Check sheet for the modelled part. Datum: model origin and axes. Units: mm. A direction names the side the tool comes from. Round coordinates to 2 decimals unless told otherwise and drop trailing zeros. Write each loop counter-clockwise with the first axis right and the second up, starting at its lowest first coordinate (ties: lowest second). Pieces come first, ordered by that corner, then holes.
Item 1: Release check for a two-part mould opening along X. For faces 1 (the flat face through (11, 143.002, 0)), 2 (the flat face through (34.355, 156.823, 9.392)), 3 (the flat face through (24, 143.002, 0)), 4 (the flat face through (18, 157, -19.05)) record: +X half, -X half, draft (parallel to the pull), parting line (faces both ways), or undercut.
Item 2: Tool access check on faces 5 (the flat face through (34.2, 156.82, -9.66)), 6 (the flat face through (31, 154.305, -8)). Record the directions out of +Z, -Z, +X, -X, +Y, -Y that give a thin tool (end or side, any length) a straight path to the whole face; none if there is none.
Item 3: Cross-section at B-B on y = 146.75. Enter the section's corners in (x, z), plus the area to 3 significant figures.
Item 4: Go/stop test with flat-tipped pins: pin 1 Ø6 at (x, y) = (4, 146.5) entering from -Z; pin 2 Ø4 at (x, y) = (6.5, 152) entering from -Z; pin 3 Ø6 at (x, y) = (3, 147) entering from -Z. Record where each tip stops, or that it passes through.
Item 5: Cross-section at A-A on x = 17.78. Enter the section's corners in (y, z) (3 decimals).
Item 6: Material ranges on line 1 (Y direction, x = 1, z = -1) (3 decimals); line 2 (Z direction, x = 24.13, y = 142.95); line 3 (X direction, y = 147.5, z = -8), recorded low to high.
from build123d import *

# Parameters (mm, degrees)
PAD012_DEPTH    = 5.08
SKETCH059_R     = 15.24
PAD013_DEPTH    = 11.43
SKETCH065_R     = 3.20675
POCKET010_DEPTH = 0.127


with BuildPart() as part:
    # Sketch058 → Pad012 (new body)
    with BuildSketch(Plane.XZ):
        Polygon((21.997045, 0), (10.998523, 19.05), (-10.998523, 19.05), (-21.997045, 0), (-10.998523, -19.05), (10.998523, -19.05), align=None)
    extrude(amount=PAD012_DEPTH)

    # Sketch059 (on Face8 of Pad012) → Pad013 (join)
    with BuildSketch(Plane.XZ.offset(5.08)):
        Circle(SKETCH059_R)
    extrude(amount=PAD013_DEPTH)

    # Sketch062 → Groove002 (revolve, cut)
    with BuildSketch(Plane.YZ):
        Polygon((-3.874167, 27.49752), (3.874167, 10.09448), (15.071476, 25.506253), align=None)
    revolve(axis=Axis((0, 0, 0), (0, 1, 0)), mode=Mode.SUBTRACT)

    # Sketch065 (on Face11 of Groove002) → Pocket010 (cut)
    with BuildSketch(Plane.XZ.offset(16.51)):
        with Locations((6.35, 0)):
            Circle(SKETCH065_R)
        with Locations((-6.35, 0)):
            Circle(SKETCH065_R)
    extrude(amount=-POCKET010_DEPTH, mode=Mode.SUBTRACT)


with BuildPart() as part_1:
    # Body009 placement: moved
    add(part.part.moved(Location((17.78, 159.385, 0))))


solid = part_1.part
Response values:
1. face 1: undercut
1. face 2: +X half
1. face 3: undercut
1. face 4: draft
2. face 5: -Z, +X, +Y, -Y
2. face 6: -Y
3. outline: circle Ø30.48 at (17.78, 0)
3. area: 730 mm2
4. pin 1: stops at z = -10.77
4. pin 2: stops at z = -12.09
4. pin 3: stops at z = -9.67
5. outline: (142.875, -15.24) - (154.305, -15.24) - (154.305, -19.05) - (159.272, -19.05) - (159.385, -18.796) - (159.385, 18.796) - (159.272, 19.05) - (154.305, 19.05) - (154.305, 15.24) - (142.875, 15.24) - close
6. line 1: y = 154.305 to 159.385
6. line 2: z = -13.85 to -3.21, 3.21 to 13.85
6. line 3: x = 4.81 to 30.75
